Geometry check sheet. Reference: the model listing, model coordinates, mm. A direction names the side the tool comes from. Coordinates: 2 decimals unless noted, no trailing zeros. Write each loop counter-clockwise with the first axis right and the second up, starting at its lowest first coordinate (ties: lowest second). Pieces come first, ordered by that corner, then holes. Notation, with made-up numbers: (68, 87.5) - (95, 87.5) arc R18 ccw to (95, 119.5) - close; hole circle Ø1 at (20.25, 58.5). An arc over 180 degrees is marked (long way). Answer as a JSON object with one key per item and string values. Group by question number.
from build123d import *

# Parameters (mm, degrees)
F1_DEPTH = 20
F2_W     = 20
F2_H     = 315
F3_DEPTH = 10
F4_SIZE2 = 184.7520861407
F4_SIZE  = 320
F5_W     = 610
F5_H     = 765
F5_W_2   = 10
F6_DEPTH = 10


with BuildPart() as f1:
    # F0 (on Front) → F1 (new body)
    with BuildSketch(Plane.XZ):
        Polygon((0, 293), (0, 0), (780, 0), (780, 315), (760, 315), (760, 10), (480, 10), (480, 305), (460, 305), (460, 10), (20, 10), (20, 293), align=None)
    extrude(amount=F1_DEPTH)

    # F2 (on face) → F3 (join)
    with BuildSketch(Plane.YZ.offset(780)):
        Polygon((-20, 0), (-20, 315), (-800, 315), (-800, -40), (0, -40), (0, 0), align=None)
        with Locations((-10, 157.5)):
            Rectangle(F2_W, F2_H)
    extrude(amount=F3_DEPTH)

    # F4
    f4_edges = [f1.edges().sort_by_distance(p)[0] for p in [
        (785, -800, 315),
    ]]
    f4_side = f1.faces().sort_by_distance((785, -800, 137.5))[0]
    chamfer(f4_edges, length=F4_SIZE, length2=F4_SIZE2, reference=f4_side)

    # F5 (on face) → F6 (join)
    with BuildSketch(Plane(origin=(0, 0, -40), x_dir=(1, 0, 0), z_dir=(0, 0, -1))):
        with Locations((475, 382.5)):
            Rectangle(F5_W, F5_H)
        with Locations((785, 382.5)):
            Rectangle(F5_W_2, F5_H)
    extrude(amount=F6_DEPTH)


solid = f1.part
(1) Set-up check for faces 1 (the face through (10, -10, 293)), 2 (the face through (476, -388, -50)), 3 (the face through (422, 0, -42)), 4 (the face through (475, -20, 112)), 5 (the face through (622, -10, 10)): record each of +Z, -Z, +X, -X, +Y, -Y from which the full face is reachable in a straight line by a thin tool's end or side.
(2) Gauge pin test, flat ends, axial feed: pin 1 (22 mm diameter, centred on x = 155, y = -9, fed in from +Z); pin 2 (8 mm diameter, centred on x = 784.5, y = -788, fed in from -Z); pin 3 (11 mm diameter, centred on y = -448, z = -45.5, fed in from -X). Record the tip position at first contact, or that the pin passes through.
(3) Section check A-A (x = 186). Record the cut outline in (y, z).
(4) Section check C-C (y = -569). Record the cut outline in (x, z), and give its area (3 significant figures).
(5) Section check B-B (z = 154). Record the cut outline in (x, y).
(6) Draft check along Z on faces 6 (the face through (0, -10, 149)), 7 (the face through (385, -10, 0)), 8 (the face through (784.93, -706.33, 157.24)). Enter one of: +Z half, -Z half, draft (parallel to the pull), parting line (faces both ways), or undercut.
(7) Section check D-D (z = 57.5). Record the cut outline in (x, y).
(8) Material ranges on L1, parallel to X at y = -667.5, z = 221; L2, parallel to Z at x = 343, y = -450.5; L3, parallel to Y at x = 479.5, z = 269.5, recorded low to high. Write a range as [from, to].
Conclusion:
{
 "1": {"face 1": "+Z, -X, +Y, -Y", "face 2": "-Z, +X, -X, +Y, -Y", "face 3": "+Z, -Z, +X, -X, +Y", "face 4": "+Z, -X, -Y", "face 5": "+Z, +Y, -Y"},
 "2": {"pin 1": "stops at z = 10", "pin 2": "stops at z = -40", "pin 3": "stops at x = 170"},
 "3": {"outline": "(-765, -50) - (0, -50) - (0, -40) - (-765, -40) - close; (-20, 0) - (0, 0) - (0, 10) - (-20, 10) - close"},
 "4": {"outline": "(170, -50) - (790, -50) - (790, 315) - (780, 315) - (780, -40) - (170, -40) - close", "area": "9,750 mm^2"},
 "5": {"outline": "(0, -20) - (20, -20) - (20, 0) - (0, 0) - close; (460, -20) - (480, -20) - (480, 0) - (460, 0) - close; (760, -20) - (780, -20) - (780, -708.2) - (790, -708.2) - (790, 0) - (760, 0) - close"},
 "6": {"face 6": "draft", "face 7": "undercut", "face 8": "+Z half"},
 "7": {"outline": "(0, -20) - (20, -20) - (20, 0) - (0, 0) - close; (460, -20) - (480, -20) - (480, 0) - (460, 0) - close; (760, -20) - (780, -20) - (780, -763.92) - (790, -763.92) - (790, 0) - (760, 0) - close"},
 "8": {"L1": "x = [780, 790]", "L2": "z = [-50, -40]", "L3": "y = [-20, 0]"}
}
